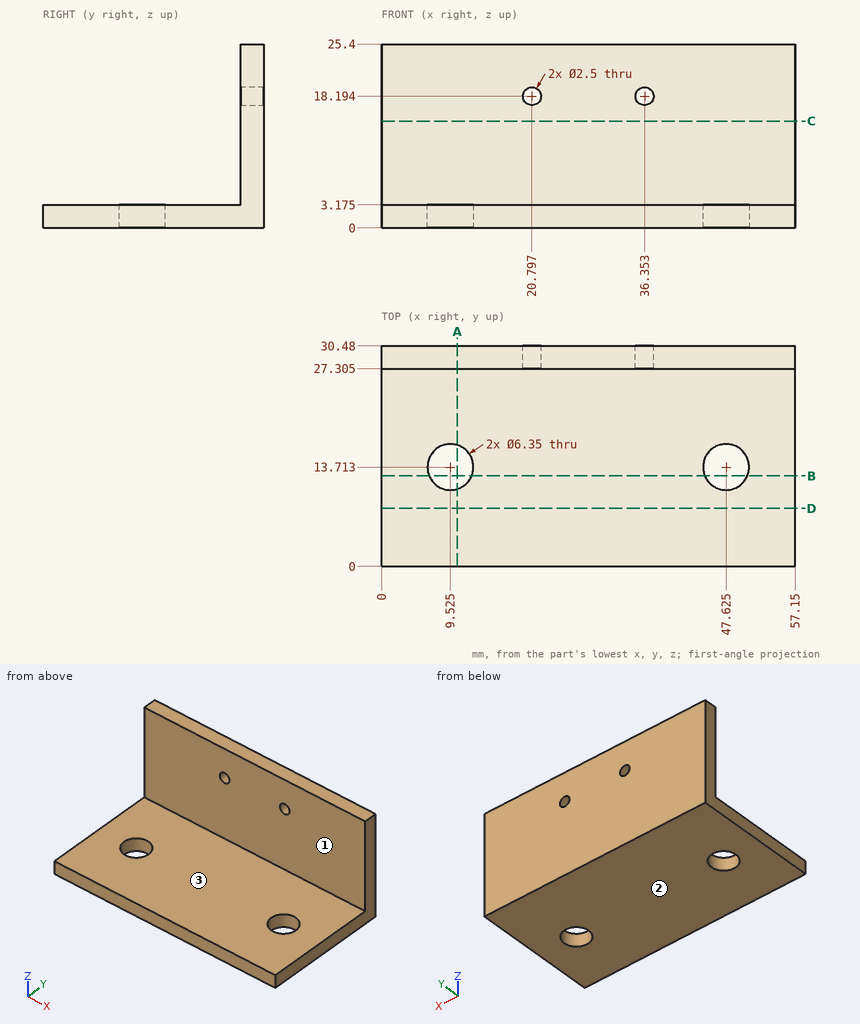
Answer from the drawing. Dimensions are ordinates in mm from the lowest x, y and z of the part. Give positions to 0.01 mm unless a question says otherwise; leave off trailing zeros. Order: outer loops, then holes, each group sorted by start corner. A loop starts at its lowest first (then second) coordinate and runs counter-clockwise, first axis right, second up. Notation, with made-up numbers: (-12, 60.25) - (9, 60.25) arc R16 cw to (9, 64.25) - close; hole circle Ø10 at (38.5, -3). An arc over 180 degrees is marked (long way). One line per item, written item: value. Start each with the question number.
1. Consider line 1 (Z direction, x = 22.5, y = 4.5) (3 decimals); line 2 (Y direction, x = 32.5, z = 15.5) (3 decimals). Determine where each line is inside the solid, lowest interval first.
2. Each of these flat-tipped pins is pushed along its axis until it touches: pin 1 Ø10 at (x, y) = (15.5, 9.5) entering from +Z (3 decimals); pin 2 Ø8 at (x, z) = (42.5, 11) entering from -Y (3 decimals). Where does it stop, or does it pass through?
3. For a pull along Z with two mould halves and no side action, classify the marked faces 1, 2 and 3 as released by +Z, released by -Z, zero draft, split by the parting line, or undercut.
4. Section C-C, the plane z = 14.75 is taken. Write down the section's boundary in (x, y) (3 decimals).
5. Section B-B, the plane y = 12.5 is taken. Count the separate pieces of the cut face and the enclosed holes in it, then the cut area to 3 significant figures.
6. Section A-A, the plane x = 10.5 is taken. Write down the section's boundary in (y, z) (1 decimal).
7. Section D-D, the plane y = 8 is taken. Write down the section's boundary in (x, z) (3 decimals).
Filled sheet:
1. line 1: 0 to 3.175
1. line 2: 27.305 to 30.48
2. pin 1: z = 3.175
2. pin 2: y = 27.305
3. face 1: zero draft
3. face 2: released by -Z
3. face 3: released by +Z
4. outline: (0, 27.305) - (57.15, 27.305) - (57.15, 30.48) - (0, 30.48) - close
5. separate pieces: 3
5. enclosed holes: 0
5. area: 144 mm²
6. outline: (0, 0) - (10.7, 0) - (10.7, 3.2) - (0, 3.2) - close; (16.7, 0) - (30.5, 0) - (30.5, 25.4) - (27.3, 25.4) - (27.3, 3.2) - (16.7, 3.2) - close
7. outline: (0, 0) - (57.15, 0) - (57.15, 3.175) - (0, 3.175) - close
